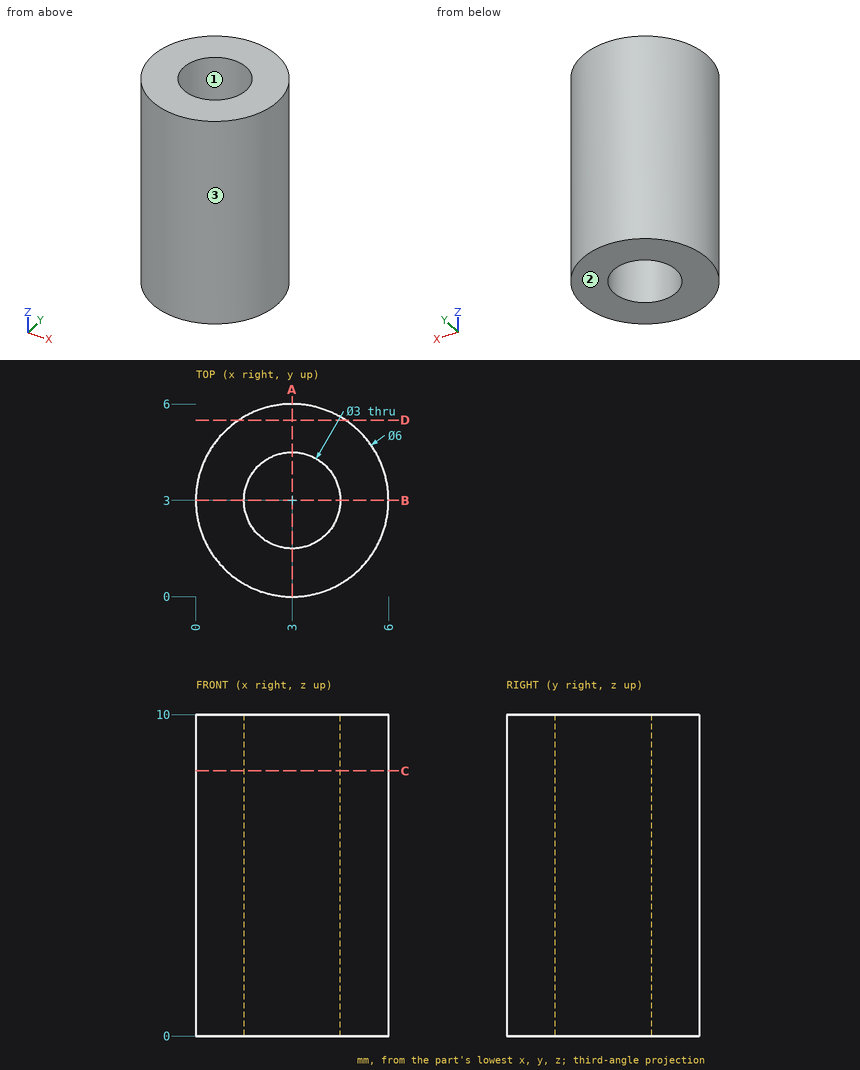
Source: three-view drawing plus pictorial views. Frame: mm from the lowest corner of the part. Round coordinates to 2 decimals unless told otherwise and drop trailing zeros. Order: outer loops, then holes, each group sorted by start corner. A loop starts at its lowest first (then second) coordinate and runs counter-clockwise, first axis right, second up. Notation, with made-up numbers: M -28.75,84.25 L -11.75,84.25 A22 cw -11.75,94.25 Z; hole C 7,65 d10. An arc over 180 degrees is marked long. One line per item, written item: value.
(1) Pull-direction query (Y, two-part tool) for the marked faces 1, 2 and 3; classes: pulls with the +Y half, pulls with the -Y half, needs draft (parallel to the pull), parting line crosses it, or undercut.
Result sheet:
face 1: undercut
face 2: needs draft
face 3: parting line crosses it
(2) Pin query (flat end, axial travel): P1, Ø1, axis at x = 2, z = 7.5, coming from the +Y side; P2, Ø1, axis at x = 5.5, z = 4.5, coming from the +Y side; P3, Ø1.5, axis at y = 1.5, z = 7.5, coming from the +X side. Return the tip coordinate at first contact, or that it passes through.
Result sheet:
P1: y = 5.96
P2: y = 5.24
P3: x = 5.9
(3) Cut plane A-A (x = 3). Return the cut outline in (y, z), and give its area (3 significant figures).
Result sheet:
outline: M 0,0 L 1.5,0 L 1.5,10 L 0,10 Z; M 4.5,0 L 6,0 L 6,10 L 4.5,10 Z
area: 30.0 mm2
(4) Cut plane C-C (z = 8.25). Return the cut outline in (x, y).
Result sheet:
outline: C 3,3 d6; hole C 3,3 d3
(5) Cut plane D-D (y = 5.5). Return the cut outline in (x, z), and give its area (3 significant figures).
Result sheet:
outline: M 1.34,0 L 4.66,0 L 4.66,10 L 1.34,10 Z
area: 33.2 mm2
(6) Line query: probe 1 along Y at (x, z) = (3, 3.25); probe 2 along X at (y, z) = (5.6, 5.25); probe 3 along Y at (x, z) = (2.1, 7.75). Output: solid intervals per line, ascending. Write a range as [from, to].
Result sheet:
probe 1: [0, 1.5], [4.5, 6]
probe 2: [1.5, 4.5]
probe 3: [0.14, 1.8], [4.2, 5.86]
